For this review, take the finished solid that the model builds, in its own axes (mm). Round coordinates to 2 decimals unless told otherwise and drop trailing zeros. Order: outer loops, then holes, each group sorted by start corner. A loop starts at its lowest first (then second) coordinate and runs counter-clockwise, first axis right, second up. Notation, with made-up numbers: (65.25, 22) - (74.25, 22) arc R24 ccw to (74.25, 32) - close; hole circle Ø9 at (-28, 53). An arc over 180 degrees is marked (long way). Write each question's results on one line, items separated by ' | '. Start each with the question number.
(1) Take a section at A-A, the plane z = 3.45. Give the boundary of the cut face in (x, y), plus the area to 3 significant figures.
(2) Insertion check: pin 1 Ø2.5 at (x, y) = (-74.61, 137.4) entering from -Z; pin 2 Ø1.4 at (x, z) = (1, 3) entering from +Y. Each pin has a flat end and moves straight along its axis. Give the tip position at first contact, or say it passes through.
(3) For L1, parallel to X at y = 121.65, z = 1.85; L2, parallel to X at y = 40, z = 2.05; L3, parallel to X at y = 137, z = 1.4, list the stretches that pass through material, from the lowest coordinate up. Write a range as from..to.
(4) Take a section at B-B, the plane y = -1. Give the boundary of the cut face in (x, z).
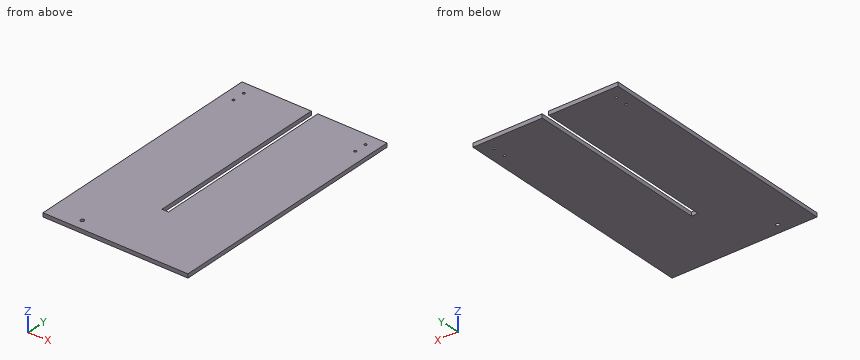
```python
from build123d import *

# Parameters (mm, degrees)
SKETCH2_W           = 4.7625
SKETCH2_H           = 44.223214285
SKETCH2_H_2         = 44.223214286
SKETCH2_W_2         = 21.998214286
SKETCH2_H_3         = 4.7625
SKETCH2_W_3         = 26.760714286
BOSS_EXTRUDE1_DEPTH = 4.7625
SKETCH3_W           = 7.9375
SKETCH3_H           = 228.6
CUT_EXTRUDE1_DEPTH  = 184.017476539
SKETCH4_R           = 2.3
CUT_EXTRUDE2_DEPTH  = 184.017476539
SKETCH5_R           = 1.5
CUT_EXTRUDE3_DEPTH  = 4.7625
SKETCH6_W           = 4.7625
SKETCH6_H           = 44.223214286
BOSS_EXTRUDE2_DEPTH = 4.7625
SKETCH7_W           = 26.760714286
SKETCH7_H           = 4.7625
CUT_EXTRUDE4_DEPTH  = 4.7625
SKETCH9_W           = 4.7625
SKETCH9_H           = 221.116071428
SKETCH9_W_2         = 21.998214286
SKETCH9_H_2         = 4.7625
CUT_EXTRUDE5_DEPTH  = 4.7625


with BuildPart() as part:
    # Sketch2 → Boss-Extrude1 (new body)
    with BuildSketch(Plane.XY):
        Polygon((0, -152.4), (0, 152.4), (-88.9, 152.4), (-88.9, 108.176785714), (-88.9, 63.953571429), (-88.9, 19.730357143), (-88.9, -24.492857143), (-88.9, -68.716071429), (-88.9, -112.939285714), (-88.9, -152.4), (-66.901785714, -152.4), (-40.141071429, -152.4), (-13.380357143, -152.4), align=None)
        Polygon((88.9, 152.4), (0, 152.4), (0, -152.4), (13.380357143, -152.4), (40.141071429, -152.4), (66.901785714, -152.4), (88.9, -152.4), (88.9, -112.939285714), (88.9, -68.716071429), (88.9, -24.492857143), (88.9, 19.730357143), (88.9, 63.953571429), (88.9, 108.176785714), align=None)
        with Locations((-91.28125, 86.065178572)):
            Rectangle(SKETCH2_W, SKETCH2_H)
        with Locations((-91.28125, -2.38125)):
            Rectangle(SKETCH2_W, SKETCH2_H_2)
        with Locations((-91.28125, -90.827678572)):
            Rectangle(SKETCH2_W, SKETCH2_H)
        with Locations((-77.900892857, -154.78125)):
            Rectangle(SKETCH2_W_2, SKETCH2_H_3)
        with Locations((-26.760714286, -154.78125)):
            Rectangle(SKETCH2_W_3, SKETCH2_H_3)
        with Locations((26.760714286, -154.78125)):
            Rectangle(SKETCH2_W_3, SKETCH2_H_3)
        with Locations((91.28125, -90.827678572)):
            Rectangle(SKETCH2_W, SKETCH2_H)
        with Locations((91.28125, -2.38125)):
            Rectangle(SKETCH2_W, SKETCH2_H_2)
        with Locations((91.28125, 86.065178572)):
            Rectangle(SKETCH2_W, SKETCH2_H)
        with Locations((77.900892857, -154.78125)):
            Rectangle(SKETCH2_W_2, SKETCH2_H_3)
    extrude(amount=BOSS_EXTRUDE1_DEPTH)

    # Sketch3 → Cut-Extrude1 (cut, through all)
    with BuildSketch(Plane.XY.offset(4.7625)):
        with Locations((0, 38.1)):
            Rectangle(SKETCH3_W, SKETCH3_H)
    extrude(amount=-CUT_EXTRUDE1_DEPTH, mode=Mode.SUBTRACT)

    # Sketch4 → Cut-Extrude2 (cut, through all)
    with BuildSketch(Plane.XY.offset(4.7625)):
        with Locations((-50.8, -139.7)):
            Circle(SKETCH4_R)
    extrude(amount=-CUT_EXTRUDE2_DEPTH, mode=Mode.SUBTRACT)

    # Sketch5 → Cut-Extrude3 (cut)
    with BuildSketch(Plane.XY.offset(4.7625)):
        with Locations((-74.6125, 137.4)):
            Circle(SKETCH5_R)
        with Locations((-74.6125, 121.65)):
            Circle(SKETCH5_R)
        with Locations((74.6125, 121.65)):
            Circle(SKETCH5_R)
        with Locations((74.6125, 137.4)):
            Circle(SKETCH5_R)
    extrude(amount=-CUT_EXTRUDE3_DEPTH, mode=Mode.SUBTRACT)

    # Sketch6 → Boss-Extrude2 (add)
    with BuildSketch(Plane.XY.offset(4.7625)):
        with Locations((-91.28125, 41.841964286)):
            Rectangle(SKETCH6_W, SKETCH6_H)
        with Locations((-91.28125, -46.604464286)):
            Rectangle(SKETCH6_W, SKETCH6_H)
        with Locations((91.28125, 41.841964286)):
            Rectangle(SKETCH6_W, SKETCH6_H)
        with Locations((91.28125, -46.604464286)):
            Rectangle(SKETCH6_W, SKETCH6_H)
    extrude(amount=-BOSS_EXTRUDE2_DEPTH)

    # Sketch7 → Cut-Extrude4 (cut)
    with BuildSketch(Plane.XY.offset(4.7625)):
        with Locations((-26.760714286, -154.78125)):
            Rectangle(SKETCH7_W, SKETCH7_H)
        with Locations((26.760714286, -154.78125)):
            Rectangle(SKETCH7_W, SKETCH7_H)
    extrude(amount=-CUT_EXTRUDE4_DEPTH, mode=Mode.SUBTRACT)

    # Sketch9 → Cut-Extrude5 (cut)
    with BuildSketch(Plane(origin=(0, 0, 0), x_dir=(-1, 0, 0), z_dir=(0, 0, -1))):
        with Locations((-91.28125, -2.38125)):
            Rectangle(SKETCH9_W, SKETCH9_H)
        with Locations((91.28125, -2.38125)):
            Rectangle(SKETCH9_W, SKETCH9_H)
        with Locations((-77.900892857, -154.78125)):
            Rectangle(SKETCH9_W_2, SKETCH9_H_2)
        with Locations((77.900892857, -154.78125)):
            Rectangle(SKETCH9_W_2, SKETCH9_H_2)
    extrude(amount=-CUT_EXTRUDE5_DEPTH, mode=Mode.SUBTRACT)


solid = part.part
```
Results below:
1) outline: (-88.9, -152.4) - (88.9, -152.4) - (88.9, 152.4) - (3.97, 152.4) - (3.97, -76.2) - (-3.97, -76.2) - (-3.97, 152.4) - (-88.9, 152.4) - close; hole circle Ø3 at (-74.61, 121.65); hole circle Ø3 at (-74.61, 137.4); hole circle Ø4.6 at (-50.8, -139.7); hole circle Ø3 at (74.61, 121.65); hole circle Ø3 at (74.61, 137.4) | area: 52,300 mm^2
2) pin 1: passes through | pin 2: stops at y = -76.2
3) L1: x = -88.9..-76.11, -73.11..-3.97, 3.97..73.11, 76.11..88.9 | L2: x = -88.9..-3.97, 3.97..88.9 | L3: x = -88.9..-76.06, -73.17..-3.97, 3.97..73.17, 76.06..88.9
4) outline: (-88.9, 0) - (-3.97, 0) - (-3.97, 4.76) - (-88.9, 4.76) - close; (3.97, 0) - (88.9, 0) - (88.9, 4.76) - (3.97, 4.76) - close
